Could you check a few things on this model? Use its own coordinates, in mm. Face numbers are marked on the shaded views. A direction names the side the tool comes from. Round coordinates to 2 decimals unless told otherwise and drop trailing zeros. Loops run counter-clockwise (first coordinate to the right, second up) from the corner with the lowest first, then second, coordinate; pieces in that order, holes last. Notation, with made-up numbers: (-5, 5) -> (39, 5) arc R21 ccw to (39, 19) -> close; hole circle Ø4 at (73, -15). An arc over 180 degrees is marked (long way). One line per item, written item: value.
```python
from build123d import *

# Parameters (mm, degrees)
SKETCH1_W           = 28
SKETCH1_H           = 40
SKETCH1_R           = 9.5
BOSS_EXTRUDE1_DEPTH = 6
SKETCH2_W           = 10
SKETCH2_H           = 6
BOSS_EXTRUDE2_DEPTH = 4
CHAMFER1_SIZE       = 2
SKETCH3_R           = 1.5
CUT_EXTRUDE1_DEPTH  = 53.687759489
SKETCH4_R           = 12.5
SKETCH4_R_2         = 3
BOSS_EXTRUDE3_DEPTH = 3
CHAMFER2_SIZE       = 1


with BuildPart() as part:
    # Sketch1 → Boss-Extrude1 (new body)
    with BuildSketch(Plane.XY):
        with Locations((14, 20)):
            Rectangle(SKETCH1_W, SKETCH1_H)
        with Locations((14, 25)):
            Circle(SKETCH1_R, mode=Mode.SUBTRACT)
    extrude(amount=BOSS_EXTRUDE1_DEPTH)

    # Sketch2 → Boss-Extrude2 (add)
    with BuildSketch(Plane(origin=(0, 0, 0), x_dir=(1, 0, 0), z_dir=(0, 1, 0))):
        with Locations((-5, -3)):
            Rectangle(SKETCH2_W, SKETCH2_H)
        with Locations((33, -3)):
            Rectangle(SKETCH2_W, SKETCH2_H)
    extrude(amount=BOSS_EXTRUDE2_DEPTH)

    # Chamfer1
    chamfer1_edges = [part.edges().sort_by_distance(p)[0] for p in [
        (0, 4, 3),
        (-10, 4, 3),
        (28, 4, 3),
        (38, 4, 3),
        (0, 40, 3),
        (28, 40, 3),
    ]]
    chamfer(chamfer1_edges, length=CHAMFER1_SIZE)

    # Sketch3 → Cut-Extrude1 (cut, through all)
    with BuildSketch(Plane(origin=(0, 4, 0), x_dir=(1, 0, 0), z_dir=(0, 1, 0))):
        with Locations(Location((-5, -3, 0), (0, 0, 270))):
            Circle(SKETCH3_R)
        with Locations(Location((33, -3, 0), (0, 0, 270))):
            Circle(SKETCH3_R)
    extrude(amount=-CUT_EXTRUDE1_DEPTH, mode=Mode.SUBTRACT)

    # Sketch4 → Boss-Extrude3 (add)
    with BuildSketch(Plane.XY.offset(6)):
        with Locations((14, 25)):
            Circle(SKETCH4_R)
        with Locations((14, 25)):
            Circle(SKETCH4_R_2, mode=Mode.SUBTRACT)
    extrude(amount=BOSS_EXTRUDE3_DEPTH)

    # Chamfer2
    chamfer2_edges = [part.edges().sort_by_distance(p)[0] for p in [
        (1.5, 25, 9),
    ]]
    chamfer(chamfer2_edges, length=CHAMFER2_SIZE)


solid = part.part
```
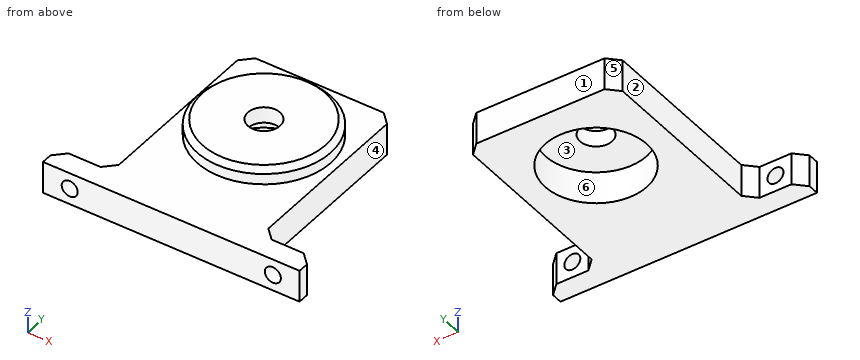
Item 1: I need wall thicknesses on line 1 (X direction, y = 1.8, z = 3); line 2 (Y direction, x = 14, z = 7.1); line 3 (X direction, y = 3.1, z = 3). Which ranges of each line are inside material? Lowest first, please. Write a range as from..to.
Output:
line 1: x = -10..-6.5, -3.5..31.5, 34.5..38
line 2: y = 12.5..22, 28..37.5
line 3: x = -8.9..-6.5, -3.5..31.5, 34.5..36.9
Item 2: For the marked faces 1 and 2, which set-ups out of +Z, -Z, +X, -X, +Y, -Y let a thin tool reach every point of the face, with its end or its side?
Output:
face 1: +Z, -Z, +X, -X, +Y
face 2: +Z, -Z, -X, +Y
Item 3: If we section it at A-A on z = 3: List the corners of the cut face in (x, y) for me.
Output:
outline: (-10, 0) -> (-6.5, 0) -> (-6.5, 4) -> (-8, 4) -> (-10, 2) -> close; (-3.5, 0) -> (31.5, 0) -> (31.5, 4) -> (30, 4) -> (28, 6) -> (28, 38) -> (26, 40) -> (2, 40) -> (0, 38) -> (0, 6) -> (-2, 4) -> (-3.5, 4) -> close; (34.5, 0) -> (38, 0) -> (38, 2) -> (36, 4) -> (34.5, 4) -> close; hole circle Ø19 at (14, 25)
Item 4: If we section it at B-B on y = 25: List the corners of the cut face in (x, z) for me, plus the area to 3 significant figures.
Output:
outline: (0, 0) -> (4.5, 0) -> (4.5, 6) -> (11, 6) -> (11, 9) -> (2.5, 9) -> (1.5, 8) -> (1.5, 6) -> (0, 6) -> close; (17, 6) -> (23.5, 6) -> (23.5, 0) -> (28, 0) -> (28, 6) -> (26.5, 6) -> (26.5, 8) -> (25.5, 9) -> (17, 9) -> close
area: 110 mm²
Item 5: If we section it at C-C on x = 14: List the corners of the cut face in (y, z) for me.
Output:
outline: (0, 0) -> (15.5, 0) -> (15.5, 6) -> (22, 6) -> (22, 9) -> (13.5, 9) -> (12.5, 8) -> (12.5, 6) -> (0, 6) -> close; (28, 6) -> (34.5, 6) -> (34.5, 0) -> (40, 0) -> (40, 6) -> (37.5, 6) -> (37.5, 8) -> (36.5, 9) -> (28, 9) -> close
Item 6: If we mould it in two halves opening along Y, with no side actions, what happens to the marked faces 3, 4, 5 and 6? For each: released by +Y, released by -Y, zero draft, split by the parting line, or undercut.
Output:
face 3: undercut
face 4: zero draft
face 5: released by +Y
face 6: undercut
Item 7: If we section it at D-D on x = -5: List the corners of the cut face in (y, z) for me, plus the area to 3 significant figures.
Output:
outline: (0, 0) -> (4, 0) -> (4, 1.5) -> (0, 1.5) -> close; (0, 4.5) -> (4, 4.5) -> (4, 6) -> (0, 6) -> close
area: 12.0 mm²
Item 8: Will these pins go through, and if not, where does the flat tip stop? pin 1 Ø2 at (x, z) = (25, 6) entering from -Y; pin 2 Ø8 at (x, y) = (14, 25) entering from -Z; pin 3 Ø3 at (x, y) = (7, 4) entering from +Z; pin 4 Ø2.5 at (x, z) = (-5, 3) entering from +Y.
Output:
pin 1: stops at y = 0
pin 2: stops at z = 6
pin 3: stops at z = 6
pin 4: passes through
